from build123d import *

# Parameters (mm, degrees)
SKETCH2_R           = 2.794
BOSS_EXTRUDE1_DEPTH = 3.556
SKETCH4_R           = 1.7526
BOSS_EXTRUDE2_DEPTH = 19.05
FILLET1_R           = 0.396875
CUT_EXTRUDE1_DEPTH  = 1.5875


with BuildPart() as part:
    # Sketch2 → Boss-Extrude1 (new body)
    with BuildSketch(Plane(origin=(0, 0, 0), x_dir=(1, 0, 0), z_dir=(0, 1, 0))):
        with Locations(Location((0, 0, 0), (0, 0, 270))):
            Circle(SKETCH2_R)
    extrude(amount=BOSS_EXTRUDE1_DEPTH)

    # Sketch4 → Boss-Extrude2 (add)
    with BuildSketch(Plane.XZ):
        with Locations(Location((0, 0, 0), (0, 0, 90))):
            Circle(SKETCH4_R)
    extrude(amount=BOSS_EXTRUDE2_DEPTH)

    # Fillet1
    fillet1_edges = [part.edges().sort_by_distance(p)[0] for p in [
        (0, 0, -2.794),
        (0, 3.556, -2.794),
    ]]
    fillet(fillet1_edges, radius=FILLET1_R)

    # Sketch5 → Cut-Extrude1 (cut)
    with BuildSketch(Plane(origin=(0, 3.556, 0), x_dir=(1, 0, 0), z_dir=(0, 1, 0))):
        Polygon((-1.374815329, 0.79375), (-1.374815329, -0.79375), (0, -1.5875), (1.374815329, -0.79375), (1.374815329, 0.79375), (0, 1.5875), align=None)
    extrude(amount=-CUT_EXTRUDE1_DEPTH, mode=Mode.SUBTRACT)


solid = part.part
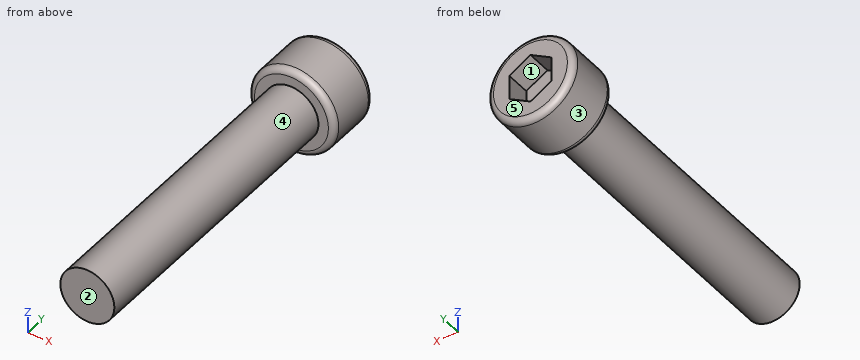
The listing builds one solid part. Answer for the finished solid, in the listing's coordinates (mm). Face numbers are marked on the shaded views. A direction names the side the tool comes from. Give positions to 0.01 mm unless a question says otherwise; leave off trailing zeros. Write each loop counter-clockwise with the first axis right and the second up, starting at its lowest first coordinate (ties: lowest second). Pieces come first, ordered by that corner, then holes.
1) Section B-B (y = -8.75) is taken. Write down the section's boundary in (x, z), and give its area (3 significant figures).
2) Section A-A (z = 0) is taken. Write down the section's boundary in (x, y), and give its area (3 significant figures).
3) Find the intervals of material crossed by L1, parallel to Y at x = -0.55, z = -0.05; L2, parallel to Y at x = 1.15, z = 1.65; L3, parallel to X at y = -17.25, z = 0.05, in increasing order.
4) A tool of negligible diameter and unlimited length cuts with its end or side. For the marked faces 4 and 5, from which of +Z, -Z, +X, -X, +Y, -Y can it reach the whole face along a straight path? Write none if from no direction.
5) Given P1, Ø1.4, axis at x = 0, z = -0.5, coming from the +Y side; P2, Ø3, axis at x = 0.5, y = -10, coming from the -Z side; P3, Ø1.5, axis at y = -10.5, z = 2, coming from the +X side, each flat-ended and moving along its own axis, determine where each tip first touches the part or whether it passes through.
6) For a pull along Z with two mould halves and no side action, classify the marked faces 1, 2 and 3 as pulls with the +Z half, pulls with the -Z half, needs draft (parallel to the pull), parting line crosses it, or undercut.
Response:
1. outline: circle Ø3.51 at (0, 0)
1. area: 9.65 mm2
2. outline: (-2.79, 0.4) arc R0.4 ccw to (-2.4, 0) - (-1.75, 0) - (-1.75, -19.05) - (1.75, -19.05) - (1.75, 0) - (2.4, 0) arc R0.4 ccw to (2.79, 0.4) - (2.79, 3.16) arc R0.4 ccw to (2.4, 3.56) - (1.37, 3.56) - (1.37, 1.97) - (-1.37, 1.97) - (-1.37, 3.56) - (-2.4, 3.56) arc R0.4 ccw to (-2.79, 3.16) - close
2. area: 82.1 mm2
3. L1: y = -19.05 to 1.97
3. L2: y = 0 to 3.56
3. L3: x = -1.75 to 1.75
4. face 4: -Y
4. face 5: +Z, -Z, +X, -X, +Y
5. P1: stops at y = 1.97
5. P2: stops at z = -1.75
5. P3: stops at x = 1.23
6. face 1: undercut
6. face 2: needs draft
6. face 3: parting line crosses it
